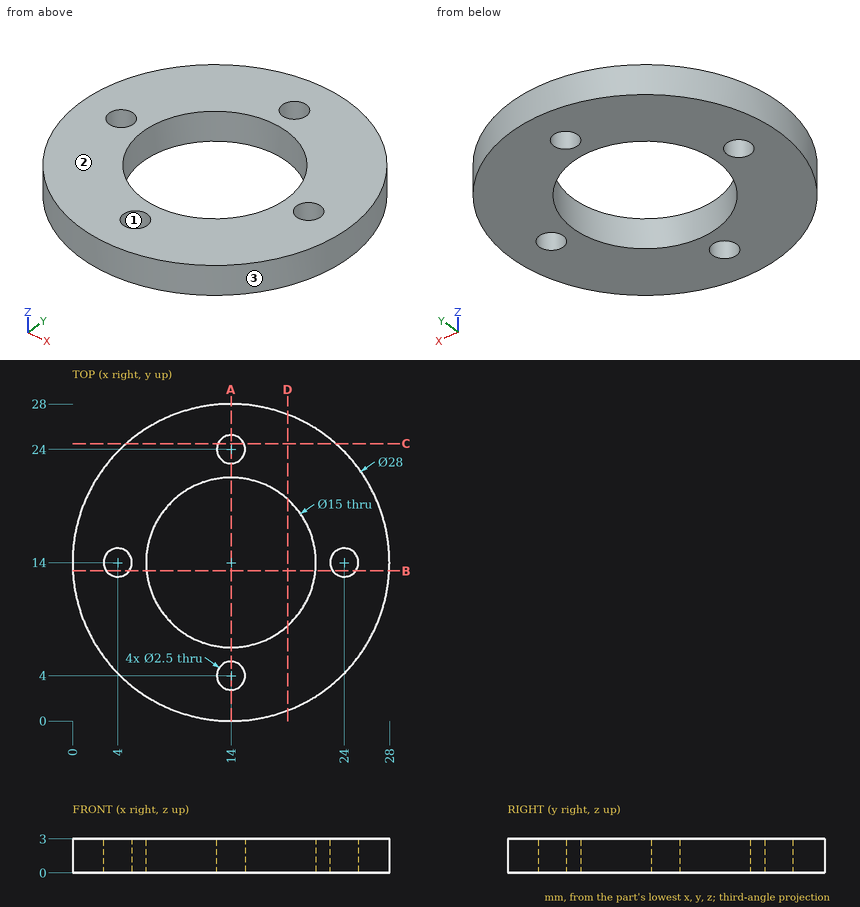
Verification items for this drawing (mm, ordinates from the low corner). Round coordinates to 2 decimals unless told otherwise and drop trailing zeros. Loops run counter-clockwise (first coordinate to the right, second up) from the corner with the lowest first, then second, coordinate; pieces in that order, holes last. Notation, with made-up numbers: (-25, 52) - (-10, 52) arc R17 ccw to (-10, 73) - close; hole circle Ø9 at (-31.5, 41). An arc over 180 degrees is marked (long way). Answer as CSV lines item,"result". Start each with the question number.
Item 1: Section check C-C (y = 24.5). Record the boundary of the cut face in (x, z), and give its area (3 significant figures).
Item 2: Release check for a two-part mould opening along Y. For the marked faces 1, 2 and 3 record: +Y half, -Y half, draft (parallel to the pull), parting line (faces both ways), or undercut.
Item 3: Section check A-A (x = 14). Record the boundary of the cut face in (y, z), and give its area (3 significant figures).
Item 4: Section check D-D (x = 19). Record the boundary of the cut face in (y, z), and give its area (3 significant figures).
Item 5: Section check B-B (y = 13.25). Record the boundary of the cut face in (x, z).
Item 6: Scan lines: line 1 (Y direction, x = 14, z = 1); line 2 (X direction, y = 10, z = 0.55); line 3 (Y direction, x = 9.25, z = 1.85). Record each from-to range of solid material in increasing order. Write a range as [from, to].
Item 7: Depth check by flat-ended pin: P1, Ø1, axis at x = 12.5, z = 2, coming from the +Y side; P2, Ø2, axis at x = 14, y = 24, coming from the +Z side. Enter the tip coordinate at first touch or a pass-through.
Report:
1,outline,"(4.74, 0) - (12.85, 0) - (12.85, 3) - (4.74, 3) - close; (15.15, 0) - (23.26, 0) - (23.26, 3) - (15.15, 3) - close"
1,area,"48.7 mm2"
2,face 1,"undercut"
2,face 2,"draft"
2,face 3,"parting line"
3,outline,"(0, 0) - (2.75, 0) - (2.75, 3) - (0, 3) - close; (5.25, 0) - (6.5, 0) - (6.5, 3) - (5.25, 3) - close; (21.5, 0) - (22.75, 0) - (22.75, 3) - (21.5, 3) - close; (25.25, 0) - (28, 0) - (28, 3) - (25.25, 3) - close"
3,area,"24.0 mm2"
4,outline,"(0.92, 0) - (8.41, 0) - (8.41, 3) - (0.92, 3) - close; (19.59, 0) - (27.08, 0) - (27.08, 3) - (19.59, 3) - close"
4,area,"44.9 mm2"
5,outline,"(0.02, 0) - (3, 0) - (3, 3) - (0.02, 3) - close; (5, 0) - (6.54, 0) - (6.54, 3) - (5, 3) - close; (21.46, 0) - (23, 0) - (23, 3) - (21.46, 3) - close; (25, 0) - (27.98, 0) - (27.98, 3) - (25, 3) - close"
6,line 1,"y = [0, 2.75], [5.25, 6.5], [21.5, 22.75], [25.25, 28]"
6,line 2,"x = [0.58, 7.66], [20.34, 27.42]"
6,line 3,"y = [0.83, 8.2], [19.8, 27.17]"
7,P1,"stops at y = 27.96"
7,P2,"passes through"
